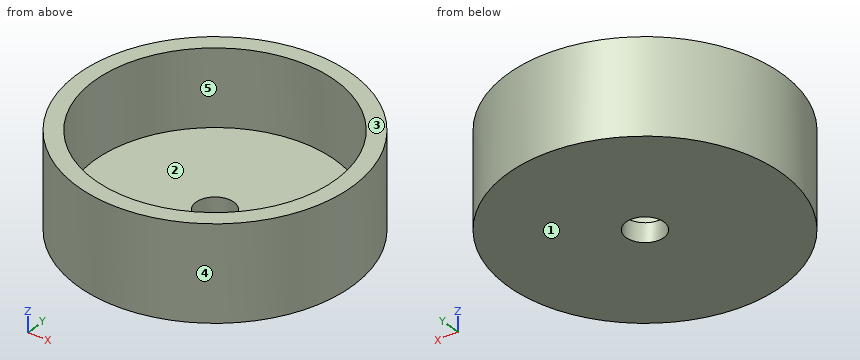
from build123d import *

# Parameters (mm, degrees)
F0_R     = 14.5
F1_DEPTH = 10
F2_R     = 12.75
F3_DEPTH = 8
F4_R     = 2
F5_DEPTH = 2


with BuildPart() as f1:
    # F0 (on Top) → F1 (new body)
    with BuildSketch(Plane.XY):
        Circle(F0_R)
    extrude(amount=F1_DEPTH)

    # F2 (on face) → F3 (cut)
    with BuildSketch(Plane.XY.offset(10)):
        Circle(F2_R)
    extrude(amount=-F3_DEPTH, mode=Mode.SUBTRACT)

    # F4 (on Top) → F5 (cut)
    with BuildSketch(Plane.XY):
        Circle(F4_R)
    extrude(amount=F5_DEPTH, mode=Mode.SUBTRACT)


solid = f1.part
Input: part model. Units: mm. Frame: model coordinates. Face numbers are marked on the shaded views. A direction names the side the tool comes from. Coordinates: 2 decimals unless noted, no trailing zeros. Loops run counter-clockwise (first coordinate to the right, second up) from the corner with the lowest first, then second, coordinate; pieces in that order, holes last. Notation, with made-up numbers: (-22, 81.25) -> (-15, 81.25) arc R34 cw to (-15, 115.25) -> close; hole circle Ø5 at (-18, -36.5). An arc over 180 degrees is marked (long way). Write each question's results on one line, items separated by ' | '. Start each with the question number.
Q1. Pin query (flat end, axial travel): pin 1 (3 mm diameter, centred on x = 6, z = 8, fed in from +Y); pin 2 (1 mm diameter, centred on x = 4.5, z = 8.5, fed in from +Y); pin 3 (6 mm diameter, centred on x = 2.5, y = -7, fed in from -Z); pin 4 (6 mm diameter, centred on x = -11, z = 7.5, fed in from -Y). Return the tip coordinate at first contact, or that it passes through.
Q2. Pull-direction query (Y, two-part tool) for the marked faces 3, 4 and 5; classes: released by +Y, released by -Y, zero draft, split by the parting line, or undercut.
Q3. Section D-D, the plane z = 2.5. Return the cut outline in (x, y).
Q4. Section A-A, the plane y = 0. Return the cut outline in (x, z).
Q5. Ray query, line 1 (Y direction, x = 0, z = 5); line 2 (Y direction, x = 0, z = 0.9); line 3 (Z direction, x = -4.25, y = -6.5). Return the intervals inside material, ascending. Write a range as from..to.
Q6. Section C-C, the plane y = 9.25. Return the cut outline in (x, z).
Q7. Reachability of the marked faces 1 and 2 from +Z, -Z, +X, -X, +Y, -Y: full face, straight path, thin tool, end or side. Return the list, or none.
Found:
1) pin 1: y = 13.78 | pin 2: y = 13.94 | pin 3: z = 0 | pin 4: y = -12.09
2) face 3: zero draft | face 4: split by the parting line | face 5: undercut
3) outline: circle Ø29 at (0, 0); hole circle Ø25.5 at (0, 0)
4) outline: (-14.5, 0) -> (-2, 0) -> (-2, 2) -> (-12.75, 2) -> (-12.75, 10) -> (-14.5, 10) -> close; (2, 0) -> (14.5, 0) -> (14.5, 10) -> (12.75, 10) -> (12.75, 2) -> (2, 2) -> close
5) line 1: -14.5..-12.75, 12.75..14.5 | line 2: -14.5..-2, 2..14.5 | line 3: 0..2
6) outline: (-11.17, 0) -> (11.17, 0) -> (11.17, 10) -> (8.77, 10) -> (8.77, 2) -> (-8.77, 2) -> (-8.77, 10) -> (-11.17, 10) -> close
7) face 1: -Z, +X, -X, +Y, -Y | face 2: +Z
